Geometry: final body of the model. Coordinates: model frame, mm. A direction names the side the tool comes from. Give positions to 0.01 mm unless a question says otherwise; leave off trailing zeros. Loops run counter-clockwise (first coordinate to the right, second up) from the corner with the lowest first, then second, coordinate; pieces in that order, holes last. Notation, with made-up numbers: (41, 85) - (97, 85) arc R21 cw to (97, 113) - close; hole circle Ø11 at (-25.5, 45.25). An arc over 180 degrees is marked (long way). Answer in a Markdown table with one row per item.
from build123d import *

# Parameters (mm, degrees)
SKETCH4_R           = 127
BOSS_EXTRUDE1_DEPTH = 254
SKETCH5_R           = 114.3
BOSS_EXTRUDE2_DEPTH = 25.4
CHAMFER1_SIZE       = 25.4


with BuildPart() as part:
    # Sketch3 → Revolve1 (revolve)
    with BuildSketch(Plane.XY, mode=Mode.PRIVATE) as revolve1_sk:
        with BuildLine():
            Line((-12.7, 177.8), (-63.5, 177.8))
            Line((-63.5, 177.8), (-63.5, 0))
            Line((-63.5, 0), (0, 0))
            ThreePointArc((0, 0), (0.183912717, 89.366708051), (-12.7, 177.8))
        make_face()
    revolve(revolve1_sk.sketch.rotate(Axis((-63.5, 0, 0), (1, 0, 0)), 90), axis=Axis((-63.5, 0, 0), (1, 0, 0)))

    # Sketch4 → Boss-Extrude1 (add)
    with BuildSketch(Plane.ZY.offset(63.5)):
        Circle(SKETCH4_R)
    extrude(amount=-BOSS_EXTRUDE1_DEPTH)

    # Sketch5 → Boss-Extrude2 (add)
    with BuildSketch(Plane(origin=(190.5, 0, 0), x_dir=(0, 0, -1), z_dir=(1, 0, 0))):
        Circle(SKETCH5_R)
    extrude(amount=BOSS_EXTRUDE2_DEPTH)

    # Chamfer1
    chamfer1_edges = [part.edges().sort_by_distance(p)[0] for p in [
        (215.9, 0, 114.3),
    ]]
    chamfer(chamfer1_edges, length=CHAMFER1_SIZE - 0.0001)  # a hair under: the kernel refuses the full size


solid = part.part
Q1. First-contact query: pin 1 (1.5 mm diameter, centred on x = 180, y = 50, fed in from +Z); pin 2 (10 mm diameter, centred on x = 3.5, y = -27, fed in from -Z); pin 3 (8 mm diameter, centred on x = 132, z = -55, fed in from -Y). Flat tips, straight axial feed; report the tip coordinate or a pass-through.
Check values:
| item | result |
|---|---|
| pin 1 | z = 117.06 |
| pin 2 | z = -125.08 |
| pin 3 | y = -116.31 |
Q2. Cut plane B-B (x = -39). Output: boundary loops of the cut face in (y, z), and give its area (3 significant figures).
Check values:
| item | result |
|---|---|
| outline | circle Ø355.6 at (0, 0) |
| area | 99,300 mm² |
Q3. Reachability of faces 1 (the cylindrical face through (92.05, -123.98, -27.53)), 2 (the flat face through (215.9, 1, 1)) from +Z, -Z, +X, -X, +Y, -Y: full face, straight path, thin tool, end or side. Return the list, or none.
Check values:
| item | result |
|---|---|
| face 1 | +X |
| face 2 | +Z, -Z, +X, +Y, -Y |
Q4. Material intervals for line 1 along X through (y, z) = (79.5, 97); line 2 along Y through (x, z) = (116, 2); line 3 along Z through (x, y) = (-45, 131), sorted ascending.
Check values:
| item | result |
|---|---|
| line 1 | -63.5 to 190.5 |
| line 2 | -126.98 to 126.98 |
| line 3 | -120.22 to 120.22 |
Q5. Cut plane A-A (x = 173). Output: boundary loops of the cut face in (y, z).
Check values:
| item | result |
|---|---|
| outline | circle Ø254 at (0, 0) |
